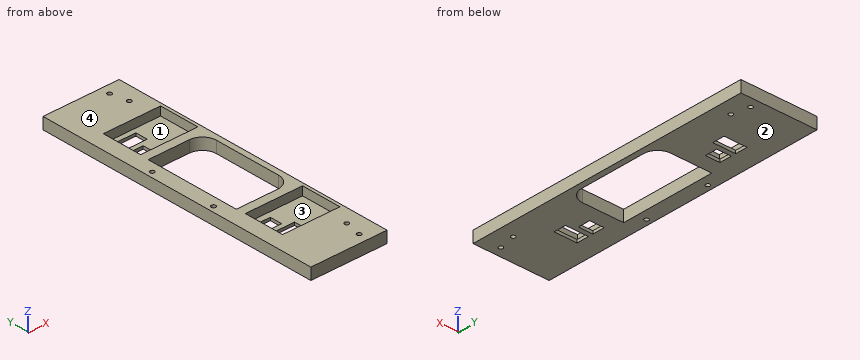
from build123d import *

# Parameters (mm, degrees)
F0_W     = 83.82
F0_H     = 317.5
F0_R     = 2.38125
F1_DEPTH = 12.7
F2_W     = 62.992
F2_H     = 44.196
F3_DEPTH = 9.525
F4_W     = 15.9385
F4_H     = 13.462
F4_W_2   = 25.2222
F5_DEPTH = 3.176


with BuildPart() as f1:
    # F0 (on Top) → F1 (new body)
    with BuildSketch(Plane.XY):
        with Locations((-41.91, 158.75)):
            Rectangle(F0_W, F0_H)
        with Locations((-77.47, 122.2502)):
            Circle(F0_R, mode=Mode.SUBTRACT)
        with Locations((-20.5994, 10.795)):
            Circle(F0_R, mode=Mode.SUBTRACT)
        with Locations((-16.637, 29.845)):
            Circle(F0_R, mode=Mode.SUBTRACT)
        with BuildLine():
            ThreePointArc((-6.3246, 121.793), (-10.840369, 110.890969), (-21.7424, 106.3752))
            Line((-21.7424, 106.3752), (-36.2458, 106.3752))
            Line((-36.2458, 106.3752), (-67.0814, 106.3752))
            Line((-67.0814, 106.3752), (-67.0814, 137.2108))
            Line((-67.0814, 137.2108), (-67.0814, 179.9844))
            Line((-67.0814, 179.9844), (-67.0814, 210.82))
            Line((-67.0814, 210.82), (-36.2458, 210.82))
            Line((-36.2458, 210.82), (-21.7424, 210.82))
            ThreePointArc((-21.7424, 210.82), (-10.840369, 206.304231), (-6.3246, 195.4022))
            Line((-6.3246, 195.4022), (-6.3246, 121.793))
        make_face(mode=Mode.SUBTRACT)
        with Locations((-77.47, 194.945)):
            Circle(F0_R, mode=Mode.SUBTRACT)
        with Locations((-16.637, 287.655)):
            Circle(F0_R, mode=Mode.SUBTRACT)
        with Locations((-20.5994, 306.705)):
            Circle(F0_R, mode=Mode.SUBTRACT)
    extrude(amount=F1_DEPTH)

    # F2 (on face) → F3 (cut)
    with BuildSketch(Plane.XY.offset(12.7)):
        with Locations((-34.798, 74.4474)):
            Rectangle(F2_W, F2_H)
        with Locations((-34.798, 242.7478)):
            Rectangle(F2_W, F2_H)
    extrude(amount=-F3_DEPTH, mode=Mode.SUBTRACT)

    # F4 (on face) → F5 (cut, through all)
    with BuildSketch(Plane.XY.offset(3.175)):
        with Locations((-52.83835, 233.934)):
            Rectangle(F4_W, F4_H)
        with Locations((-48.1965, 252.603)):
            Rectangle(F4_W_2, F4_H)
        with Locations((-52.83835, 83.2612)):
            Rectangle(F4_W, F4_H)
        with Locations((-48.1965, 64.5922)):
            Rectangle(F4_W_2, F4_H)
    extrude(amount=-F5_DEPTH, mode=Mode.SUBTRACT)


solid = f1.part
Verification items for the finished model (mm, model axes). Face numbers are marked on the shaded views. A direction names the side the tool comes from. Give positions to 0.01 mm unless a question says otherwise; leave off trailing zeros. Loops run counter-clockwise (first coordinate to the right, second up) from the corner with the lowest first, then second, coordinate; pieces in that order, holes last. Notation, with made-up numbers: (52.25, 71.5) - (60.25, 71.5) arc R33 ccw to (60.25, 99.5) - close; hole circle Ø5 at (23.25, 13). An arc over 180 degrees is marked (long way). Write item = value, one per line. Start each with the question number.
Q1. Tool access check on the marked faces 1 and 2. Record the directions out of +Z, -Z, +X, -X, +Y, -Y that give a thin tool (end or side, any length) a straight path to the whole face; none if there is none.
Q2. Cross-section at B-B, the plane x = -40. Enter the section's corners in (y, z) (3 decimals).
Q3. Depth check by flat-ended pin: P1, Ø4, axis at x = -16.637, y = 287.655, coming from the +Z side; P2, Ø10, axis at x = -55.5, y = 246, coming from the +Z side (3 decimals). Enter the tip coordinate at first touch or a pass-through.
Q4. Cross-section at A-A, the plane y = 253. Enter the section's corners in (x, z) (3 decimals), and give its area (3 significant figures).
Q5. Mould release check, pull along X, two halves, no side actions. Record for the marked faces 3 and 4: released by +X, released by -X, zero draft, split by the parting line, or undercut.
Q6. Thickness scan on line 1 (Y direction, x = -42, z = 10.75); line 2 (Y direction, x = -77.47, z = 7); line 3 (X direction, y = 141.5, z = 4.75). Record the ranges inside material, lowest first.
Q7. Cross-section at C-C, the plane z = 10.5. State how many separate pieces and enclosed holes the cut face has, and give its area (3 significant figures).
Q8. Cross-section at D-D, the plane x = -26. Enter the section's corners in (y, z) (3 decimals), and give its area (3 significant figures).
Answer key:
q1.face_1 = +Z
q1.face_2 = -Z, +X, -X, +Y, -Y
q2.outline = (0, 0) - (57.861, 0) - (57.861, 3.175) - (52.349, 3.175) - (52.349, 12.7) - (0, 12.7) - close; (71.323, 0) - (106.375, 0) - (106.375, 12.7) - (96.545, 12.7) - (96.545, 3.175) - (71.323, 3.175) - close; (210.82, 0) - (245.872, 0) - (245.872, 3.175) - (220.65, 3.175) - (220.65, 12.7) - (210.82, 12.7) - close; (259.334, 0) - (317.5, 0) - (317.5, 12.7) - (264.846, 12.7) - (264.846, 3.175) - (259.334, 3.175) - close
q3.P1 = through
q3.P2 = 3.175
q4.outline = (-83.82, 0) - (-60.808, 0) - (-60.808, 3.175) - (-66.294, 3.175) - (-66.294, 12.7) - (-83.82, 12.7) - close; (-35.585, 0) - (0, 0) - (0, 12.7) - (-3.302, 12.7) - (-3.302, 3.175) - (-35.585, 3.175) - close
q4.area = 384 mm^2
q5.face_3 = undercut
q5.face_4 = zero draft
q6.line_1 = 0 to 52.35, 96.55 to 106.38, 210.82 to 220.65, 264.85 to 317.5
q6.line_2 = 0 to 119.87, 124.63 to 192.56, 197.33 to 317.5
q6.line_3 = -83.82 to -67.08, -6.32 to 0
q7.separate_pieces = 1
q7.enclosed_holes = 9
q7.area = 14,700 mm^2
q8.outline = (0, 0) - (106.375, 0) - (106.375, 12.7) - (96.545, 12.7) - (96.545, 3.175) - (52.349, 3.175) - (52.349, 12.7) - (0, 12.7) - close; (210.82, 0) - (317.5, 0) - (317.5, 12.7) - (264.846, 12.7) - (264.846, 3.175) - (220.65, 3.175) - (220.65, 12.7) - (210.82, 12.7) - close
q8.area = 1,860 mm^2
